Check sheet for the modelled part. Datum: model origin and axes. Units: mm. Face numbers are marked on the shaded views. A direction names the side the tool comes from. Give positions to 0.01 mm unless a question says otherwise; leave off trailing zeros. Loops run counter-clockwise (first coordinate to the right, second up) from the corner with the lowest first, then second, coordinate; pieces in that order, holes last. Notation, with made-up numbers: (43, 35) - (78, 35) arc R23 ccw to (78, 47) - close; hole circle Ø10 at (23.25, 2.25). An arc over 180 degrees is marked (long way). Answer in a Markdown table with one row per item. Add a question column.
(1) Sectioned sample at B-B on z = -41.5. Enter the section's corners in (x, y), then the cut area to 3 significant figures.
(2) Sectioned sample at A-A on y = 0.5. Enter the section's corners in (x, z), then the cut area to 3 significant figures.
(3) Go/stop test with flat-tipped pins: P1, Ø5, axis at x = 2.5, z = -36.5, coming from the -Y side; P2, Ø15.5, axis at y = -3.5, z = -32, coming from the -X side; P3, Ø4, axis at x = -5.5, y = 12, coming from the -Z side. Record where each tip stops, or that it passes through.
(4) Set-up check for the marked faces 1, 2 and 3: record each of +Z, -Z, +X, -X, +Y, -Y from which the full face is reachable in a straight line by a thin tool's end or side.
(5) Thickness scan on L1, parallel to Z at x = 2, y = 21.5. Record the ranges inside material, lowest first.
(6) Sectioned sample at C-C on x = -8. Enter the section's corners in (y, z) (3 decimals), then the cut area to 3 significant figures.
from build123d import *

# Parameters (mm, degrees)
SKETCH1_W           = 33
SKETCH1_H           = 63
SKETCH1_W_2         = 4.466715852
SKETCH1_H_2         = 14.293859793
BOSS_EXTRUDE1_DEPTH = 60
SKETCH1_3_W         = 4.466715852
SKETCH1_3_H         = 14.293859793
BOSS_EXTRUDE2_DEPTH = 60


with BuildPart() as part:
    # Sketch1 → Boss-Extrude1 (new body)
    # profile 1 of 2: a face of its own
    with BuildSketch(Plane.XY):
        with Locations((0, -5.625)):
            Rectangle(SKETCH1_W, SKETCH1_H)
        with Locations((2.233357926, -3.23810571)):
            Rectangle(SKETCH1_W_2, SKETCH1_H_2, mode=Mode.SUBTRACT)
    # profile 2 of 2: a face of its own
    with BuildSketch(Plane.XY):
        with Locations((2.233357926, -3.23810571)):
            Rectangle(SKETCH1_W_2, SKETCH1_H_2)
    extrude(amount=BOSS_EXTRUDE1_DEPTH)

    # Sketch1_3 → Boss-Extrude2 (add)
    with BuildSketch(Plane.XY):
        with Locations((2.233357926, -3.23810571)):
            Rectangle(SKETCH1_3_W, SKETCH1_3_H)
    extrude(amount=-BOSS_EXTRUDE2_DEPTH)


solid = part.part
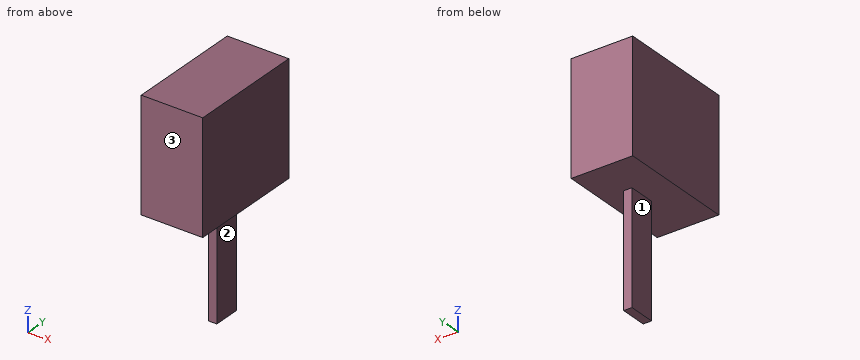
Reply:
| question | item | result |
|---|---|---|
| 1 | outline | (0, -10.39) - (4.47, -10.39) - (4.47, 3.91) - (0, 3.91) - close |
| 1 | area | 63.8 mm^2 |
| 2 | outline | (-16.5, 0) - (0, 0) - (0, -60) - (4.47, -60) - (4.47, 0) - (16.5, 0) - (16.5, 60) - (-16.5, 60) - close |
| 2 | area | 2,250 mm^2 |
| 3 | P1 | y = -10.39 |
| 3 | P2 | x = 0 |
| 3 | P3 | z = 0 |
| 4 | face 1 | -Z, -X, +Y, -Y |
| 4 | face 2 | -Z, +X, +Y, -Y |
| 4 | face 3 | +Z, -Z, +X, -X, -Y |
| 5 | L1 | 0 to 60 |
| 6 | outline | (-37.125, 0) - (25.875, 0) - (25.875, 60) - (-37.125, 60) - close |
| 6 | area | 3,780 mm^2 |
